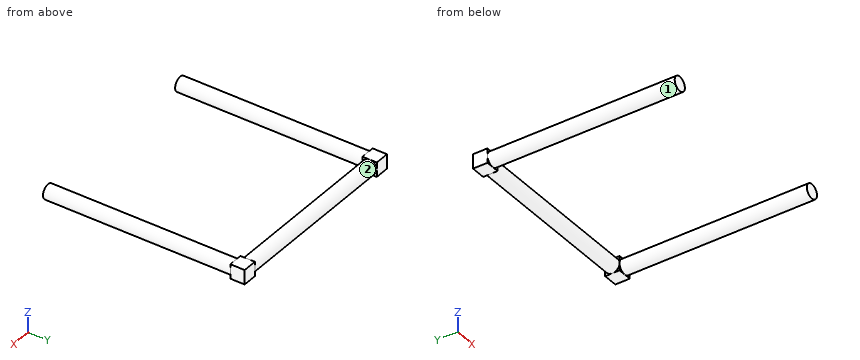
```python
from build123d import *

# Parameters (mm, degrees)
F0_R     = 12.7
F1_DEPTH = 152.4
F2_W     = 25.4
F2_H     = 25.4
F3_DEPTH = 25.4
F4_R     = 12.688144
F5_DEPTH = 330.2


with BuildPart() as f1:
    # F0 (on Right) → F1 (new body)
    with BuildSketch(Plane.YZ):
        Circle(F0_R)
    extrude(amount=-F1_DEPTH)

    # F2 (on face) → F3 (join)
    with BuildSketch(Plane(origin=(-152.4, 0, 0), x_dir=(0, -1, 0), z_dir=(-1, 0, 0))):
        Rectangle(F2_W, F2_H)
    extrude(amount=F3_DEPTH)

    # F4 (on face) → F5 (join)
    with BuildSketch(Plane.XZ.offset(12.7)):
        with Locations((-165.1, 0)):
            Circle(F4_R)
    extrude(amount=F5_DEPTH)

    # F6: F1 across face


with BuildPart() as f1_1:
    add(f1.part)
    add(f1.part.mirror(Plane.YZ))


solid = f1_1.part
```
Check sheet for the modelled part. Datum: model origin and axes. Units: mm. Face numbers are marked on the shaded views. A direction names the side the tool comes from. Round coordinates to 2 decimals unless told otherwise and drop trailing zeros. Loops run counter-clockwise (first coordinate to the right, second up) from the corner with the lowest first, then second, coordinate; pieces in that order, holes last. Notation, with made-up numbers: (9, 73) -> (27, 73) arc R21 ccw to (27, 81) -> close; hole circle Ø6 at (16, 59.5). An arc over 180 degrees is marked (long way). Answer in a Markdown table with one row per item.
Q1. Sectioned sample at B-B on z = 7.75. Enter the section's corners in (x, y), then the cut area to 3 significant figures.
Data:
| item | result |
|---|---|
| outline | (-177.8, -12.7) -> (-175.15, -12.7) -> (-175.15, -342.9) -> (-155.05, -342.9) -> (-155.05, -12.7) -> (-152.4, -12.7) -> (-152.4, -10.06) -> (152.4, -10.06) -> (152.4, -12.7) -> (155.05, -12.7) -> (155.05, -342.9) -> (175.15, -342.9) -> (175.15, -12.7) -> (177.8, -12.7) -> (177.8, 12.7) -> (152.4, 12.7) -> (152.4, 10.06) -> (-152.4, 10.06) -> (-152.4, 12.7) -> (-177.8, 12.7) -> close |
| area | 20,700 mm^2 |
Q2. Go/stop test with flat-tipped pins: P1, Ø4, axis at x = 94.5, z = -3, coming from the -Y side; P2, Ø5, axis at x = 108, z = 1.5, coming from the +Y side; P3, Ø10, axis at y = -96.5, z = -8, coming from the +X side; P4, Ø4, axis at y = -163, z = 1, coming from the +X side. Record where each tip stops, or that it passes through.
Data:
| item | result |
|---|---|
| P1 | stops at y = -12.66 |
| P2 | stops at y = 12.7 |
| P3 | stops at x = 177.43 |
| P4 | stops at x = 177.79 |
Q3. Sectioned sample at C-C on x = -88.5. Enter the section's corners in (y, z), then the cut area to 3 significant figures.
Data:
| item | result |
|---|---|
| outline | circle Ø25.4 at (0, 0) |
| area | 507 mm^2 |
Q4. Thickness scan on L1, parallel to X at y = -96, z = -2.75; L2, parallel to X at y = -284, z = 6; L3, parallel to Y at x = 64.5, z = -1.25. Record the ranges inside material, lowest first.
Data:
| item | result |
|---|---|
| L1 | x = -177.49 to -152.71, 152.71 to 177.49 |
| L2 | x = -176.28 to -153.92, 153.92 to 176.28 |
| L3 | y = -12.64 to 12.64 |
Q5. Set-up check for the marked faces 1 and 2: record each of +Z, -Z, +X, -X, +Y, -Y from which the full face is reachable in a straight line by a thin tool's end or side.
Data:
| item | result |
|---|---|
| face 1 | -Y |
| face 2 | none |
Q6. Sectioned sample at A-A on y = -269. Enter the section's corners in (x, z), then the cut area to 3 significant figures.
Data:
| item | result |
|---|---|
| outline | circle Ø25.38 at (-165.1, 0); circle Ø25.38 at (165.1, 0) |
| area | 1,010 mm^2 |
